```python
from build123d import *

# Parameters (mm, degrees)
SKETCH1_W           = 20.1
SKETCH1_H           = 20.1
BOSS_EXTRUDE1_DEPTH = 10
BOSS_EXTRUDE2_DEPTH = 8.15
SKETCH4_R           = 3.07
CUT_EXTRUDE1_DEPTH  = 34.725991461
SKETCH5_R           = 2.84
BOSS_EXTRUDE3_DEPTH = 2.2
FILLET1_R           = 1
SKETCH6_R           = 2.675
CUT_EXTRUDE2_DEPTH  = 5.15
SKETCH7_R           = 1.3
BOSS_EXTRUDE4_DEPTH = 0.5


with BuildPart() as part:
    # Sketch1 → Boss-Extrude1 (new body)
    with BuildSketch(Plane(origin=(0, 0, 0), x_dir=(1, 0, 0), z_dir=(0, 1, 0))):
        with Locations((-10.05, 10.05)):
            Rectangle(SKETCH1_W, SKETCH1_H)
    extrude(amount=BOSS_EXTRUDE1_DEPTH)

    # Sketch2 → Boss-Extrude2 (add)
    with BuildSketch(Plane(origin=(0, 10, 0), x_dir=(1, 0, 0), z_dir=(0, 1, 0))):
        Polygon((-8.177760508, 18), (-12.178797874, 18), (-14.179316556, 14.535), (-12.178797874, 11.07), (-8.177760508, 11.07), (-6.177241825, 14.535), align=None)
    extrude(amount=BOSS_EXTRUDE2_DEPTH)

    # Sketch3 → Cut-Revolve1 (revolve, cut)
    with BuildSketch(Plane(origin=(0, 0, -14.535), x_dir=(-1, 0, 0), z_dir=(0, 0, -1)), mode=Mode.PRIVATE) as cut_revolve1_sk:
        Polygon((10.278279191, 18.15), (14.179316556, 14.5), (16.20190306, 12.607569847), (16.20190306, 19.465321923), (10.278279191, 19.465321923), align=None)
    revolve(cut_revolve1_sk.sketch.rotate(Axis((-10.178279191, 18.15, -14.535), (0, 1, 0)), 270), axis=Axis((-10.178279191, 18.15, -14.535), (0, 1, 0)), mode=Mode.SUBTRACT)

    # Sketch4 → Cut-Extrude1 (cut, through all)
    with BuildSketch(Plane(origin=(0, 0, 0), x_dir=(0, 0, -1), z_dir=(1, 0, 0))):
        with Locations((5, 5)):
            Circle(SKETCH4_R)
    extrude(amount=-CUT_EXTRUDE1_DEPTH, mode=Mode.SUBTRACT)

    # Sketch5 → Boss-Extrude3 (add)
    with BuildSketch(Plane.ZY):
        with Locations((-14.3, 4.16)):
            Circle(SKETCH5_R)
    extrude(amount=-BOSS_EXTRUDE3_DEPTH)

    # Fillet1
    fillet1_edges = [part.edges().sort_by_distance(p)[0] for p in [
        (2.2, 4.16, -17.14),
    ]]
    fillet(fillet1_edges, radius=FILLET1_R)

    # Sketch6 → Cut-Extrude2 (cut)
    with BuildSketch(Plane.XZ):
        with Locations(Location((-10.178279191, -14.535, 0), (0, 0, 270))):
            Circle(SKETCH6_R)
    extrude(amount=-CUT_EXTRUDE2_DEPTH, mode=Mode.SUBTRACT)

    # Sketch7 → Boss-Extrude4 (add)
    with BuildSketch(Plane(origin=(0, 10, 0), x_dir=(1, 0, 0), z_dir=(0, 1, 0))):
        with Locations(Location((-10, 5.7, 0), (0, 0, 270))):
            Circle(SKETCH7_R)
    extrude(amount=BOSS_EXTRUDE4_DEPTH)


solid = part.part
```
Part model, mm, in its own coordinate system. A direction names the side the tool comes from. Round coordinates to 2 decimals unless told otherwise and drop trailing zeros. Loops run counter-clockwise (first coordinate to the right, second up) from the corner with the lowest first, then second, coordinate; pieces in that order, holes last.
1. Slice it at D-D (y = 8.5). Give the cut face in (x, z), and give its area (3 significant figures).
Solutions:
outline: (-20.1, -20.1) - (0, -20.1) - (0, 0) - (-20.1, 0) - close
area: 404 mm2
2. Slice it at B-B (x = -5.5). Give the cut face in (y, z).
Solutions:
outline: (0, -20.1) - (10, -20.1) - (10, 0) - (0, 0) - close; hole circle Ø6.14 at (5, -5)
3. Slice it at C-C (z = -5.7). Give the cut face in (x, y), and give its area (3 significant figures).
Solutions:
outline: (-20.1, 0) - (0, 0) - (0, 2.01) - (-20.1, 2.01) - close; (-20.1, 7.99) - (0, 7.99) - (0, 10) - (-8.7, 10) - (-8.7, 10.5) - (-11.3, 10.5) - (-11.3, 10) - (-20.1, 10) - close
area: 82.1 mm2
4. Drill centre lines: line 1 along Z through (x, y) = (-11.5, 4); line 2 along Y through (x, z) = (-14.25, -5); line 3 along X through (y, z) = (5.25, -18.5). Where is each one in solid material? Low to high.
Solutions:
line 1: z = -20.1 to -16.86, -12.21 to -7.9, -2.1 to 0
line 2: y = 0 to 1.93, 8.07 to 10
line 3: x = -20.1 to 0
5. Two-plate mould, pull along Y, no slides. Class faces 1 (the face through (-10, 0, -10)), 2 (the face through (-10, 10, -10)), 3 (the face through (-9.91, 5.92, -7.93)): pulls with the +Y half, pulls with the -Y half, needs draft (parallel to the pull), parting line crosses it, or undercut.
Solutions:
face 1: pulls with the -Y half
face 2: pulls with the +Y half
face 3: undercut
6. Flat gauge pins, fed straight in: pin 1 (3 mm diameter, centred on y = 15, z = -12.5, fed in from +X); pin 2 (10 mm diameter, centred on x = -17, z = -7.5, fed in from +Y); pin 3 (1.5 mm diameter, centred on y = 11.5, z = -5.5, fed in from -X); pin 4 (1.2 mm diameter, centred on x = -9.5, y = 12, fed in from -Z). Where does each tip first touch, or does it go through?
Solutions:
pin 1: stops at x = -6.5
pin 2: stops at y = 10
pin 3: passes through
pin 4: stops at z = -18
7. 3-axis set-ups, long thin cutter, end or side, ignore diameter. For faces 4 (the face through (0.592, 4.285, -17.137)), 5 (the face through (-13.193, 12.466, -12.827)), 6 (the face through (-13.165, 12.466, -16.292)): which of +Z, -Z, +X, -X, +Y, -Y reach the whole face in a straight line?
Solutions:
face 4: +X
face 5: +Z, -X, +Y
face 6: -Z, -X, +Y
8. Slice it at A-A (z = -3). Give the cut face in (x, y).
Solutions:
outline: (-20.1, 0) - (0, 0) - (0, 2.67) - (-20.1, 2.67) - close; (-20.1, 7.33) - (0, 7.33) - (0, 10) - (-20.1, 10) - close
